Verification items for the finished model (mm, model axes). A direction names the side the tool comes from. Give positions to 0.01 mm unless a question says otherwise; leave off trailing zeros. Order: outer loops, then holes, each group sorted by start corner. A loop starts at its lowest first (then second) coordinate and runs counter-clockwise, first axis right, second up. Notation, with made-up numbers: (49, 5) - (91, 5) arc R33 cw to (91, 38) - close; hole circle Ø1 at (39.5, 42.5). An arc over 180 degrees is marked (long way). Answer as a JSON object with one key per item and string values.
```python
from build123d import *

# Parameters (mm, degrees)
SKETCH006_R                = 2.75
PAD003_DEPTH               = 5
SKETCH006_MIRRORED003_2_R  = 2.75
PAD003_MIRRORED003_2_DEPTH = 5
BOX_W                      = 32.75
BOX_H                      = 5
BOX_DEPTH                  = 5
SKETCH007_W                = 28.75
SKETCH007_H                = 24
SKETCH007_R                = 2.5
PAD004_DEPTH               = 5
SKETCH007_MIRRORED006_2_W  = 28.75
SKETCH007_MIRRORED006_2_H  = 24
SKETCH007_MIRRORED006_2_R  = 2.5
PAD004_MIRRORED006_2_DEPTH = 5
PAD005_DEPTH               = 5
SKETCH009_R                = 1.375
PAD006_DEPTH               = 5


with BuildPart() as part:
    # Sketch006 → Pad003 (new body)
    with BuildSketch(Plane(origin=(0, 0, 30), x_dir=(1, 0, 0), z_dir=(0, -1, 0))):
        with BuildLine():
            ThreePointArc((19.5, 0), (13.788582, 13.788582), (0, 19.5))
            Line((0, 19.5), (0, 30))
            Line((28.75, 30), (0, 30))
            Line((28.75, 30), (28.75, 0))
            Line((19.5, 0), (28.75, 0))
        make_face()
        with Locations((23.5, 23.5)):
            Circle(SKETCH006_R, mode=Mode.SUBTRACT)
    pad003 = extrude(amount=PAD003_DEPTH)

    # Sketch006 Mirrored003 2 → Pad003 Mirrored003 2 (add)
    with BuildSketch(Plane(origin=(0, 0, 30), x_dir=(-1, 0, 0), z_dir=(0, 1, 0))):
        with BuildLine():
            ThreePointArc((19.5, 0), (13.788582, 13.788582), (0, 19.5))
            Line((0, 19.5), (0, 30))
            Line((28.75, 30), (0, 30))
            Line((28.75, 30), (28.75, 0))
            Line((19.5, 0), (28.75, 0))
        make_face()
        with Locations((23.5, 23.5)):
            Circle(SKETCH006_MIRRORED003_2_R, mode=Mode.SUBTRACT)
    pad003_mirrored003_2 = extrude(amount=-PAD003_MIRRORED003_2_DEPTH)

    # Mirrored004: Pad003, Pad003 Mirrored003 2 across Sketch006 H_Axis
    add(pad003.mirror(Plane(origin=(0, 0, 30), x_dir=(0, -1, 0), z_dir=(0, 0, 1))))
    add(pad003_mirrored003_2.mirror(Plane(origin=(0, 0, 30), x_dir=(0, -1, 0), z_dir=(0, 0, 1))))

    # Box → Box (join)
    with BuildSketch(Plane(origin=(0, -5, -5), x_dir=(1, 0, 0), z_dir=(0, 0, 1))):
        with Locations((16.375, 2.5)):
            Rectangle(BOX_W, BOX_H)
    box = extrude(amount=BOX_DEPTH)

    # Mirrored005: Box across YZ
    add(box.mirror(Plane.YZ))

    # Sketch007 → Pad004 (join)
    with BuildSketch(Plane(origin=(0, -29, 0), x_dir=(1, 0, 0), z_dir=(0, 0, 1))):
        with Locations((14.375, 12)):
            Rectangle(SKETCH007_W, SKETCH007_H)
        with Locations((18, 16)):
            Circle(SKETCH007_R, mode=Mode.SUBTRACT)
    pad004 = extrude(amount=-PAD004_DEPTH)

    # Sketch007 Mirrored006 2 → Pad004 Mirrored006 2 (add)
    with BuildSketch(Plane(origin=(0, -29, 0), x_dir=(-1, 0, 0), z_dir=(0, 0, -1))):
        with Locations((14.375, 12)):
            Rectangle(SKETCH007_MIRRORED006_2_W, SKETCH007_MIRRORED006_2_H)
        with Locations((18, 16)):
            Circle(SKETCH007_MIRRORED006_2_R, mode=Mode.SUBTRACT)
    pad004_mirrored006_2 = extrude(amount=PAD004_MIRRORED006_2_DEPTH)

    # Mirrored007: Pad004, Pad004 Mirrored006 2 across Sketch007 H_Axis
    add(pad004.mirror(Plane.ZX.offset(-29)))
    add(pad004_mirrored006_2.mirror(Plane.ZX.offset(-29)))

    # Sketch008 → Pad005 (join)
    with BuildSketch(Plane.YZ.offset(28.75)):
        with BuildLine():
            Line((0, 60), (-5, 60))
            add(Edge.make_bspline(
                [(-5, 60), (-53, 48.806333), (-53, 0)],
                knots=[1.802205, 1.802205, 1.802205, 3.141593, 3.141593, 3.141593], degree=2, weights=[1, 0.784012, 1]))
            Line((-53, 0), (-53, -5))
            Line((-53, -5), (0, -5))
            Line((0, -5), (0, 60))
        make_face()
    pad005 = extrude(amount=PAD005_DEPTH)

    # Mirrored008: Pad005 across YZ
    add(pad005.mirror(Plane.YZ))

    # Sketch009 → Pad006 (join)
    with BuildSketch(Plane.XY):
        Polygon((28.75, -72), (28.75, -53), (0, -53), (0, -72), (0, -89), (28.75, -89), (28.75, -80.5), align=None)
        with Locations((24.75, -80.5)):
            Circle(SKETCH009_R, mode=Mode.SUBTRACT)
        with Locations((16.75, -80.5)):
            Circle(SKETCH009_R, mode=Mode.SUBTRACT)
    extrude(amount=-PAD006_DEPTH)


solid = part.part
```
(1) Section check C-C (x = 24.75). Record the cut outline in (y, z) (3 decimals), then the cut area to 3 significant figures.
Computed values:
{"outline": "(-89, -5) - (-81.875, -5) - (-81.875, 0) - (-89, 0) - close; (-79.125, -5) - (0, -5) - (0, 4.051) - (-5, 4.051) - (-5, 0) - (-79.125, 0) - close; (-5, 8.949) - (0, 8.949) - (0, 51.051) - (-5, 51.051) - close; (-5, 55.949) - (0, 55.949) - (0, 60) - (-5, 60) - close", "area": "682 mm²"}
(2) Material ranges on line 1 along Y through (x, z) = (-18, -3.2); line 2 along Z through (x, y) = (23.5, -3.7); line 3 along Y through (x, z) = (24.75, -1.4) (3 decimals), recorded low to high. Write a range as [from, to].
Computed values:
{"line 1": "y = [-53, -47.5], [-42.5, -15.5], [-10.5, 0]", "line 2": "z = [-5, 3.75], [9.25, 50.75], [56.25, 60]", "line 3": "y = [-89, -81.875], [-79.125, 0]"}
(3) Section check A-A (x = -23.5). Record the cut outline in (y, z), then the cut area to 3 significant figures.
Computed values:
{"outline": "(-53, -5) - (0, -5) - (0, 3.75) - (-5, 3.75) - (-5, 0) - (-53, 0) - close; (-5, 9.25) - (0, 9.25) - (0, 50.75) - (-5, 50.75) - close; (-5, 56.25) - (0, 56.25) - (0, 60) - (-5, 60) - close", "area": "510 mm²"}
(4) Section check B-B (x = 16.75). Record the cut outline in (y, z) (3 decimals), then the cut area to 3 significant figures.
Computed values:
{"outline": "(-89, -5) - (-81.875, -5) - (-81.875, 0) - (-89, 0) - close; (-79.125, -5) - (-47.165, -5) - (-47.165, 0) - (-79.125, 0) - close; (-42.835, -5) - (-15.165, -5) - (-15.165, 0) - (-42.835, 0) - close; (-10.835, -5) - (0, -5) - (0, 20.016) - (-5, 20.016) - (-5, 0) - (-10.835, 0) - close; (-5, 39.984) - (0, 39.984) - (0, 60) - (-5, 60) - close", "area": "588 mm²"}
(5) Section check D-D (z = 53.5). Count the separate pieces of the cut face and the enclosed holes in it, then the cut area to 3 significant figures.
Computed values:
{"separate pieces": "3", "enclosed holes": "0", "area": "449 mm²"}
(6) Release check for a two-part mould opening along Y. For faces 4 (the flat face through (31, -53, -2)), 5 (the flat face through (6, -37, 0)), 6 (the cylindrical face through (16, -14.5, -2.5)) record: pulls with the +Y half, pulls with the -Y half, needs draft (parallel to the pull), parting line crosses it, or undercut.
Computed values:
{"face 4": "pulls with the -Y half", "face 5": "needs draft", "face 6": "undercut"}
(7) Gauge pin test, flat ends, axial feed: pin 1 Ø12 at (x, z) = (-15.5, 26) entering from -Y; pin 2 Ø3.5 at (x, z) = (-23.5, 6.5) entering from +Y; pin 3 Ø1 at (x, y) = (4.5, -14.5) entering from +Z; pin 4 Ø1.5 at (y, z) = (-77, -2) entering from -X. Record the tip position at first contact, or that the pin passes through.
Computed values:
{"pin 1": "stops at y = -5", "pin 2": "passes through", "pin 3": "stops at z = 0", "pin 4": "stops at x = 0"}
(8) Access from +Z, -Z, +X, -X, +Y, -Y to the whole of each face (thin tool, end or side, straight path). Record for faces 1 (the flat face through (28.75, -71, -2)), 2 (the flat face through (28.75, -24, 24)), 3 (the flat face through (-17, -53, -2)).
Computed values:
{"face 1": "+Z, -Z, +X, -Y", "face 2": "+Z, -Y", "face 3": "+Z, -Z, -X, -Y"}
